Study the drawing (mm; zero at the part's minimum x, y, z) and answer. Give positions to 0.01 mm unless a question says otherwise; leave off trailing zeros. Order: outer loops, then holes, each group sorted by start corner. A loop starts at its lowest first (then second) coordinate and runs counter-clockwise, first axis right, second up. Notation, with made-up numbers: (-28, -15) - (-4, -15) arc R12 ccw to (-4, -5) - close; hole circle Ø9 at (49.5, 54). An arc over 180 degrees is marked (long way). Return JSON: item names as keys, results as strings.
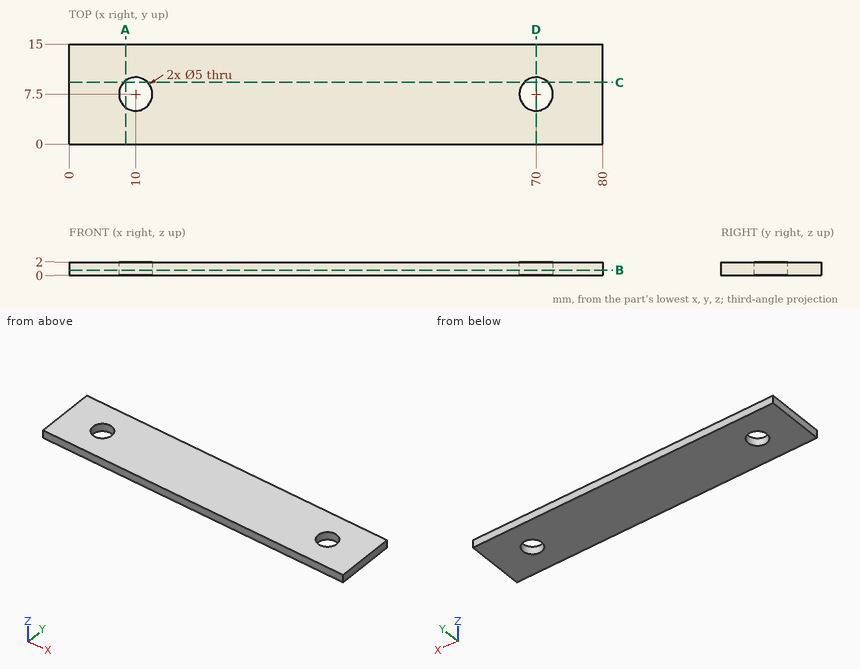
Q1. A cutting plane is placed at D-D (x = 70). Write down the section's boundary in (y, z).
Values:
{"outline": "(0, 0) - (5, 0) - (5, 2) - (0, 2) - close; (10, 0) - (15, 0) - (15, 2) - (10, 2) - close"}
Q2. A cutting plane is placed at B-B (z = 0.8). Write down the section's boundary in (x, y), and give its area (3 significant figures).
Values:
{"outline": "(0, 0) - (80, 0) - (80, 15) - (0, 15) - close; hole circle Ø5 at (10, 7.5); hole circle Ø5 at (70, 7.5)", "area": "1,160 mm²"}
Q3. Given pin 1 (5 mm diameter, centred on x = 71, y = 4, fed in from -Z), flat-ended and moving along its own axis, determine where the tip first touches the part or whether it passes through.
Values:
{"pin 1": "stops at z = 0"}
Q4. A cutting plane is placed at A-A (x = 8.5). Write down the section's boundary in (y, z), and give its area (3 significant figures).
Values:
{"outline": "(0, 0) - (5.5, 0) - (5.5, 2) - (0, 2) - close; (9.5, 0) - (15, 0) - (15, 2) - (9.5, 2) - close", "area": "22.0 mm²"}
Q5. Consider L1, parallel to Y at x = 70, z = 0.85; L2, parallel to X at y = 9.5, z = 1.6; L3, parallel to X at y = 9.75, z = 1.45. Determine where each line is inside the solid, lowest interval first.
Values:
{"L1": "y = 0 to 5, 10 to 15", "L2": "x = 0 to 8.5, 11.5 to 68.5, 71.5 to 80", "L3": "x = 0 to 8.91, 11.09 to 68.91, 71.09 to 80"}
Q6. A cutting plane is placed at C-C (y = 9.25). Write down the section's boundary in (x, z), and give its area (3 significant figures).
Values:
{"outline": "(0, 0) - (8.21, 0) - (8.21, 2) - (0, 2) - close; (11.79, 0) - (68.21, 0) - (68.21, 2) - (11.79, 2) - close; (71.79, 0) - (80, 0) - (80, 2) - (71.79, 2) - close", "area": "146 mm²"}
